Could you check a few things on this model? Use its own coordinates, in mm. A direction names the side the tool comes from. Give positions to 0.01 mm unless a question says otherwise; leave off trailing zeros. Loops run counter-clockwise (first coordinate to the right, second up) from the corner with the lowest first, then second, coordinate; pieces in that order, holes last. Notation, with made-up numbers: (80.25, 54) - (87.25, 54) arc R27 ccw to (87.25, 86) - close; hole circle Ø11 at (87.5, 35.5). An arc over 180 degrees is marked (long way). One line per item, written item: value. Start each with the question number.
Q1. If I drill on line 1 (Y direction, x = 0, z = 30), over which ranges is the centre line in solid material (lowest first)? Write a range as from..to.
Q2. If we mould it in two halves opening along Y, with no side actions, what happens to faces 3 (the face through (-9.3, 50, -6.2)), 4 (the face through (-2.38, 10.74, 32.76)), 5 (the face through (12.932, 33.238, 5.362)), 6 (the face through (12.932, 5.362, 32.762))? For each: released by +Y, released by -Y, zero draft, split by the parting line, or undercut.
Q3. I'm going to push flat-ended pins straight in: P1, Ø3, axis at x = 3.5, z = 14.5, coming from the -Y side; P2, Ø13, axis at x = 0, z = 0, coming from the -Y side; P3, Ø10, axis at y = -7, z = -1.5, coming from the -X side. Where does each tip first touch, or does it pass through?
Q4. I want a section at D-D (x = 4.5). Please give me the cut outline in (y, z).
Q5. I want a section at B-B (y = 18). Please give me the cut outline in (x, z), then the cut area to 3 significant figures.
Q6. For faces 1 (the face through (-2.38, 33.24, 10.74)), 2 (the face through (6.2, -9.3, 50)), which set-ups out of +Z, -Z, +X, -X, +Y, -Y let a thin tool reach every point of the face, with its end or its side?
Q7. I want a section at A-A (x = 0). Please give me the cut outline in (y, z).
Autodesk Inventor part; units mm, degrees
ref_plane "Work Plane1" through (0, 0, 50) normal (0, 0, 1) x (1, 0, 0)
ref_plane "Work Plane2" through (0, 50, 0) normal (0, 1, 0) x (-1, 0, 0)
ref_plane "YZ Plane" through (0, 0, 0) normal (1, 0, 0) x (0, 1, 0)
ref_plane "Work Plane1" through (0, 0, 50) normal (0, 0, 1) x (1, 0, 0)
sketch "Sketch1" plane through (0, 0, 50) normal (0, 0, 1) x (1, 0, 0)
  circle A0 centre (0, 0) radius 14
  dimension "d1" = 28
ref_plane "Work Plane2" through (0, 50, 0) normal (0, 1, 0) x (-1, 0, 0)
sketch "Sketch2" plane through (0, 50, 0) normal (0, 1, 0) x (-1, 0, 0)
  circle A0 centre (0, 0) radius 14
  dimension "d3" = 28
sketch "Sketch3" plane through (0, 0, 0) normal (1, 0, 0) x (0, 1, 0)
  line L0 (50, -14) -> (50, 14) construction
  line L1 (14, 50) -> (-14, 50) construction
  line L2 (50, 0) -> (0, 0)
  line L3 (0, 50) -> (0, 0)
  line L4 (14, 50) -> (14, 16)
  line L5 (16, 14) -> (50, 14)
  arc A0 (14, 16) -> (16, 14) centre (16, 16) ccw
  dimension "d4" = 2
sweep "Sweep1" add profiles "Sketch1" path "Sketch3" path curves L4 A0 L5
shell "Shell1" thickness 3 removed faces 2 at (7.0627, 50, -5.5585) at (0.1834, -3.0946, 50)
properties part number "90º Elbow"
Worked answers:
1. line 1: y = -14..-11, 11..14
2. face 3: released by +Y
2. face 4: undercut
2. face 5: zero draft
2. face 6: split by the parting line
3. P1: stops at y = -13.83
3. P2: stops at y = -12.46
3. P3: stops at x = -11.56
4. outline: (-13.26, 16) arc R29.26 ccw to (16, -13.26) - (50, -13.26) - (50, -10.04) - (16, -10.04) arc R26.04 cw to (-10.04, 16) - (-10.04, 50) - (-13.26, 50) - close; (10.04, 16) arc R5.96 ccw to (16, 10.04) - (50, 10.04) - (50, 13.26) - (16, 13.26) arc R2.74 cw to (13.26, 16) - (13.26, 50) - (10.04, 50) - close
5. outline: circle Ø28 at (0, 0); hole circle Ø22 at (0, 0)
5. area: 236 mm²
6. face 1: +Y
6. face 2: +Z, +X, -X, +Y, -Y
7. outline: (-14, 16) arc R30 ccw to (16, -14) - (50, -14) - (50, -11) - (16, -11) arc R27 cw to (-11, 16) - (-11, 50) - (-14, 50) - close; (11, 16) arc R5 ccw to (16, 11) - (50, 11) - (50, 14) - (16, 14) arc R2 cw to (14, 16) - (14, 50) - (11, 50) - close
